Input: part model. Units: mm. Frame: model coordinates. Face numbers are marked on the shaded views. Round coordinates to 2 decimals unless told otherwise and drop trailing zeros. Order: outer loops, then holes, each group sorted by start corner. A loop starts at its lowest first (then second) coordinate and runs counter-clockwise, first axis right, second up. Notation, with made-up numbers: (1, 36) -> (10, 36) arc R30 ccw to (10, 59) -> close; hole circle Ø7 at (54, -15.5). An arc over 180 degrees is marked (long way). Use a Markdown table: item, result.
Autodesk Inventor part; units mm, degrees
ref_plane "YZ Plane" through (0, 0, 0) normal (1, 0, 0) x (0, 1, 0)
ref_plane "XZ Plane" through (0, 0, 0) normal (0, 1, 0) x (-1, 0, 0)
ref_plane "XY Plane" through (0, 0, 0) normal (0, 0, 1) x (1, 0, 0)
sketch "Sketch1" plane through (0, 0, 0) normal (0, 1, 0) x (-1, 0, 0)
  circle A0 centre (0, 0) radius 11.375
  circle A1 centre (0, 0) radius 20
  circle A2 centre (0, 0) radius 18.25
  dimension "d0" = 22.75
  dimension "d1" = 40
  dimension "d2" = 36.5
extrude "Extrusion1" add sketch "Sketch1" along normal blind 12.25 contours A0 | A1 | A2
extrude "Extrusion2" cut sketch "Sketch1" along normal blind 6 contours A1 | A2
sketch "Sketch2" plane through (0, 0, 0) normal (1, 0, 0) x (0, 1, 0)
  line L0 (6, -20) -> (6, 20)
  line L1 (12.25, -20) -> (12.25, 20)
  line L2 (6, 20) -> (12.25, 20)
  line L3 (12.25, -20) -> (8.25, -20)
  line L4 (8.25, -20) -> (8.25, 20)
  line L5 (8.25, 20) -> (12.25, 20)
  line L6 (12.25, 20) -> (12.25, -20)
  arc A0 (8.25, -20) -> (8.25, 20) centre (-69.846, 0) ccw
  line L7 (-50.15, 0) -> (22.65, 0)
  line L8 (6, -20) -> (6, 20)
  line L9 (6, 11.375) -> (6, -11.375)
  line L10 (0, 11.375) -> (0, -11.375)
  line L11 (6, 11.375) -> (12.25, 11.375)
  line L12 (12.25, 11.375) -> (12.25, -11.375)
  line L13 (12.25, -11.375) -> (6, -11.375)
  line L14 (6, -11.375) -> (6, 11.375)
  line L15 (0, 11.375) -> (12.25, 11.375)
  line L16 (12.25, 11.375) -> (12.25, -11.375)
  line L17 (12.25, -11.375) -> (0, -11.375)
  line L18 (0, -11.375) -> (0, 11.375)
  line L19 (8.25, 18.5) -> (6, 18.5)
  line L20 (6, 18.5) -> (6, -18.5)
  line L21 (6, -18.5) -> (8.25, -18.5)
  line L22 (8.25, -18.5) -> (8.25, 18.5)
  arc A1 (7.9022, -19.9109) -> (8.25, 18.5) centre (-69.846, 0) ccw
  point P0 (12.25, 0)
  point P1 (6, 0)
  point P2 (8.25, 0)
  point P3 (10.7703, 0)
  point P4 (12.25, 0)
  point P5 (9.6011, 11.375)
  dimension "d8" = 4
revolve "Revolution1" cut sketch "Sketch2" angle 360 about axis through (0, -10, 0) along (0, 1, 0) contours L0 L19 L4 L11 | L4 A1 L11 | A0 L11 L1 L7 | A0 L2 L1 L11
sketch "Sketch3" plane through (0, 0, 0) normal (0, -1, 0) x (1, 0, 0)
  circle A0 centre (0, 0) radius 11.375
hole "Hole1" at (0, 0, 0) direction (0, 1, 0) diameter 17.1881 depth 5
properties part number "E-Stop Button" material "ABS Plastic"
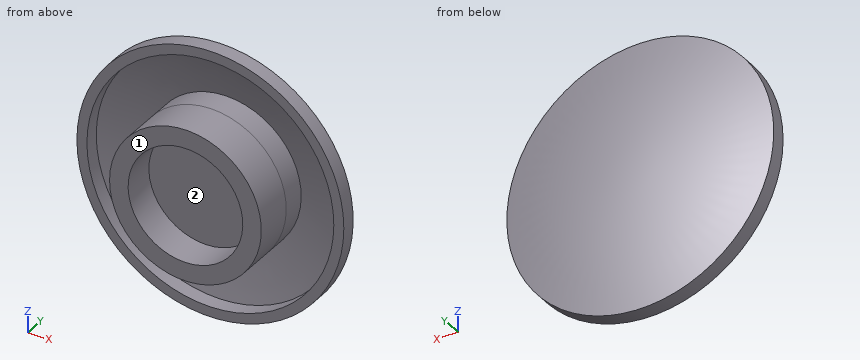
1) Line query: L1, parallel to X at y = 6.5, z = 0 (3 decimals); L2, parallel to X at y = 3.4, z = 0 (3 decimals). Output: solid intervals per line, ascending. Write a range as [from, to].
Results found:
| item | result |
|---|---|
| L1 | x = [-20, -18.5], [-11.375, 11.375], [18.5, 20] |
| L2 | x = [-11.375, -8.594], [8.594, 11.375] |
2) Pull-direction query (Z, two-part tool) for the marked faces 1 and 2; classes: +Z half, -Z half, draft (parallel to the pull), parting line (faces both ways), or undercut.
Results found:
| item | result |
|---|---|
| face 1 | draft |
| face 2 | undercut |
3) Cut plane B-B on y = 5.5. Return loops of the section in (x, z) (3 decimals).
Results found:
| item | result |
|---|---|
| outline | circle Ø22.75 at (0, 0) |
4) Pin query (flat end, axial travel): pin 1 Ø2 at (y, z) = (3, 9) entering from +X; pin 2 Ø3 at (y, z) = (5, 2) entering from +X; pin 3 Ø3 at (y, z) = (3.5, 3) entering from +X. Return the tip coordinate at first contact, or that it passes through.
Results found:
| item | result |
|---|---|
| pin 1 | stops at x = 8.09 |
| pin 2 | stops at x = 19.98 |
| pin 3 | stops at x = 11.28 |
5) Cut plane A-A on y = 1.25. Return loops of the section in (x, z) (3 decimals), and give its area (3 significant figures).
Results found:
| item | result |
|---|---|
| outline | circle Ø22.75 at (0, 0); hole circle Ø17.188 at (0, 0) |
| area | 174 mm² |
